from build123d import *

# Parameters (mm, degrees)
EXTRUDE1_DEPTH = 33.274


with BuildPart() as part:
    # Sketch1 → Extrude1 (new body)
    with BuildSketch(Plane(origin=(0, 0, 0), x_dir=(1, 0, 0), z_dir=(0, 1, 0))):
        with BuildLine():
            Line((-46.765869926, 36.668915011), (-46.765869926, -22.186880092))
            ThreePointArc((-46.765869926, -22.186880092), (-45.277972374, -25.778982541), (-41.685869926, -27.266880092))
            Line((-41.685869926, -27.266880092), (17.169925177, -27.266880092))
            ThreePointArc((17.169925177, -27.266880092), (21.863233202, -24.130911929), (20.762027626, -18.594777644))
            Line((20.762027626, -18.594777644), (-38.093767478, 40.261017459))
            ThreePointArc((-38.093767478, 40.261017459), (-43.629901762, 41.362223036), (-46.765869926, 36.668915011))
        make_face()
        with BuildLine():
            Line((-42.955869926, 36.668915011), (-42.955869926, -22.186880092))
            ThreePointArc((-42.955869926, -22.186880092), (-42.583895538, -23.084905705), (-41.685869926, -23.456880092))
            Line((-41.685869926, -23.456880092), (17.169925177, -23.456880092))
            ThreePointArc((17.169925177, -23.456880092), (18.343252183, -22.672888052), (18.067950789, -21.28885448))
            Line((18.067950789, -21.28885448), (-40.787844314, 37.566940623))
            ThreePointArc((-40.787844314, 37.566940623), (-42.171877885, 37.842242017), (-42.955869926, 36.668915011))
        make_face(mode=Mode.SUBTRACT)
    extrude(amount=EXTRUDE1_DEPTH)


solid = part.part
Geometry: final body of the model. Coordinates: model frame, mm. A direction names the side the tool comes from. Coordinates: 2 decimals unless noted, no trailing zeros. Loops run counter-clockwise (first coordinate to the right, second up) from the corner with the lowest first, then second, coordinate; pieces in that order, holes last. Notation, with made-up numbers: (-19, -29) - (35, -29) arc R17 cw to (35, -22) - close; hole circle Ø1 at (32, -8.5). An arc over 180 degrees is marked (long way). One line per question, with ' | ' between items. Start each with the question number.
(1) Draft query along X for faces 3 (the cylindrical face through (18.335, 16.404, 22.692)), 4 (the cylindrical face through (-45.317, 16.404, 25.739)), 5 (the cylindrical face through (-42.15, 16.4, -37.85)), 6 (the flat face through (-15, 0, -13)). Return one class per face: +X half, -X half, draft (parallel to the pull), parting line (faces both ways), or undercut.
(2) Cut plane B-B on z = -8. Output: boundary loops of the cut face in (x, y), and give its area (3 significant figures).
(3) Reachability of faces 1 (the flat face through (-10.95, 16.4, -7.73)), 2 (the flat face through (-13, 16, 27.267)) from +Z, -Z, +X, -X, +Y, -Y: full face, straight path, thin tool, end or side. Return the list, or none.
(4) Cut plane C-C on x = -13. Output: boundary loops of the cut face in (y, z).
(5) Ray query, L1, parallel to X at y = 24, z = -22.5; L2, parallel to Z at x = -27, y = 30; L3, parallel to X at y = 17, z = 10. Return the intervals inside material, ascending. Write a range as from..to.
(6) Cut plane A-A on y = 13.5. Output: boundary loops of the cut face in (x, z).
(7) First-contact query: pin 1 (1.5 mm diameter, centred on x = -9.5, y = 23.5, fed in from -Z); pin 2 (12 mm diameter, centred on x = -29.5, y = 9.5, fed in from -Z); pin 3 (1 mm diameter, centred on y = 13, z = -2, fed in from +X). Flat tips, straight axial feed; report the tip coordinate or a pass-through.
Here are the results:
1) face 3: undercut | face 4: -X half | face 5: undercut | face 6: draft
2) outline: (-46.77, 0) - (-42.96, 0) - (-42.96, 33.27) - (-46.77, 33.27) - close; (-11.22, 0) - (-5.83, 0) - (-5.83, 33.27) - (-11.22, 33.27) - close | area: 306 mm²
3) face 1: +Y, -Y | face 2: +Z, +X, -X, +Y, -Y
4) outline: (0, -15.17) - (33.27, -15.17) - (33.27, -9.78) - (0, -9.78) - close; (0, 23.46) - (33.27, 23.46) - (33.27, 27.27) - (0, 27.27) - close
5) L1: -46.77..-42.96, -25.72..-20.33 | L2: -29.17..-23.78, 23.46..27.27 | L3: -46.77..-42.96, 6.78..12.17
6) outline: (-46.77, -36.67) arc R5.08 ccw to (-38.09, -40.26) - (20.76, 18.59) arc R5.08 ccw to (17.17, 27.27) - (-41.69, 27.27) arc R5.08 ccw to (-46.77, 22.19) - close; hole (-42.96, -36.67) arc R1.27 ccw to (-40.79, -37.57) - (18.07, 21.29) arc R1.27 ccw to (17.17, 23.46) - (-41.69, 23.46) arc R1.27 ccw to (-42.96, 22.19) - close
7) pin 1: z = -12.42 | pin 2: z = -37.67 | pin 3: x = 0.67
